from build123d import *

# Parameters (mm, degrees)
F0_W     = 150
F0_H     = 150
F0_W_2   = 5
F0_H_2   = 5
F1_DEPTH = 10
F3_R     = 2.5
F4_DEPTH = 25
F5_W     = 150
F5_H     = 10
F5_R     = 2.5
F6_DEPTH = 15


# Not quite as in the source:
# - a feature of the source that left no trace in its solid (it failed there, or was rolled back) is left out


with BuildPart() as f1:
    # F0 (on Top) → F1 (new body)
    with BuildSketch(Plane.XY):
        Rectangle(F0_W, F0_H)
        Rectangle(F0_W_2, F0_H_2, mode=Mode.SUBTRACT)
    extrude(amount=F1_DEPTH)

    # F3 (on face) → F4 (join)
    with BuildSketch(Plane.YZ.offset(75)):
        Polygon((75, 0), (75, 10), (-75, 10), (-75, 0), (0, 0), align=None)
        with Locations((-50, 5)):
            Circle(F3_R, mode=Mode.SUBTRACT)
        with Locations((50, 5)):
            Circle(F3_R, mode=Mode.SUBTRACT)
    extrude(amount=F4_DEPTH)

    # F5 (on face) → F6 (join)
    with BuildSketch(Plane(origin=(-75, 0, 0), x_dir=(0, -1, 0), z_dir=(-1, 0, 0))):
        with Locations((0, 5)):
            Rectangle(F5_W, F5_H)
        with Locations((-50, 5)):
            Circle(F5_R, mode=Mode.SUBTRACT)
        with Locations((50, 5)):
            Circle(F5_R, mode=Mode.SUBTRACT)
    extrude(amount=F6_DEPTH)


solid = f1.part
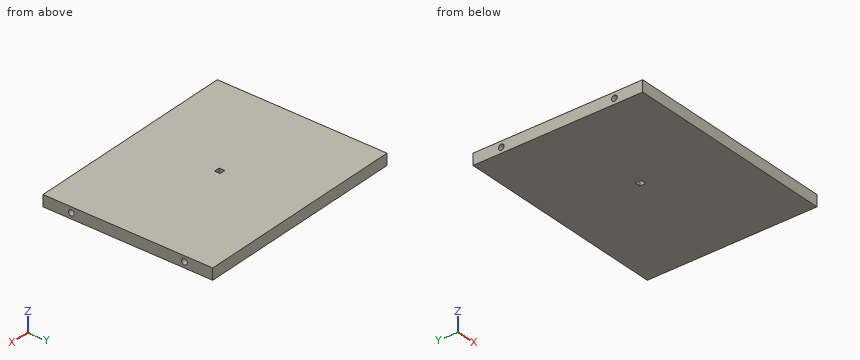
Read the model definition and answer for the solid it produces. Units are mm, in the model's axes. Coordinates: 2 decimals unless noted, no trailing zeros. Order: outer loops, then holes, each group sorted by start corner. A loop starts at its lowest first (then second) coordinate and runs counter-clockwise, first axis right, second up. Notation, with made-up numbers: (-3.75, -23) -> (39.25, -23) arc R28 ccw to (39.25, 9) -> close; hole circle Ø10 at (-3, -26). An arc over 180 degrees is marked (long way). Answer as a JSON object with one key per item and string values.
1) A cutting plane is placed at A-A, the plane y = 0. Determine the outline of the cut face in (x, z).
Model answer:
{"outline": "(-90, 0) -> (-2.5, 0) -> (-2.5, 10) -> (-90, 10) -> close; (2.5, 0) -> (100, 0) -> (100, 10) -> (2.5, 10) -> close"}
2) This flat-tipped pin is pushed along its axis until it touches: pin 1 (4.5 mm diameter, centred on y = 50, z = 5, fed in from -X). Where does it stop, or does it pass through?
Model answer:
{"pin 1": "stops at x = -75"}
3) A cutting plane is placed at B-B, the plane y = 50. Determine the outline of the cut face in (x, z), plus the area to 3 significant figures.
Model answer:
{"outline": "(-90, 0) -> (100, 0) -> (100, 2.5) -> (75, 2.5) -> (75, 7.5) -> (100, 7.5) -> (100, 10) -> (-90, 10) -> (-90, 7.5) -> (-75, 7.5) -> (-75, 2.5) -> (-90, 2.5) -> close", "area": "1,700 mm²"}
4) Consider line 1 along X through (y, z) = (-1, 8.5); line 2 along Z through (x, y) = (-78.25, 50). Determine where each line is inside the solid, lowest interval first. Write a range as from..to.
Model answer:
{"line 1": "x = -90..-2.5, 2.5..100", "line 2": "z = 0..2.5, 7.5..10"}
